```python
from build123d import *

# Parameters (mm, degrees)
RESSALTO_EXTRUS_O1_DEPTH = 15
ESBO_O2_R                = 2.5
CORTE_EXTRUS_O1_DEPTH    = 126.770027202
ESBO_O3_R                = 2.5
CORTE_EXTRUS_O2_DEPTH    = 35.768628391


with BuildPart() as part:
    # Esboço1 → Ressalto-extrusão1 (new body)
    with BuildSketch(Plane.XY):
        with BuildLine():
            Line((98.783276764, -3.569201676), (98.783276764, 17.230798324))
            ThreePointArc((98.783276764, 17.230798324), (99.369063202, 18.645011887), (100.783276764, 19.230798324))
            Line((100.783276764, 19.230798324), (121.583276764, 19.230798324))
            ThreePointArc((121.583276764, 19.230798324), (122.290383546, 19.523691543), (122.583276764, 20.230798324))
            Line((122.583276764, 20.230798324), (122.583276764, 20.430798324))
            Line((122.583276764, 20.430798324), (97.583276764, 20.430798324))
            Line((97.583276764, 20.430798324), (97.583276764, -4.569201676))
            Line((97.583276764, -4.569201676), (97.783276764, -4.569201676))
            ThreePointArc((97.783276764, -4.569201676), (98.490383546, -4.276308457), (98.783276764, -3.569201676))
        make_face()
    extrude(amount=RESSALTO_EXTRUS_O1_DEPTH)

    # Esboço2 → Corte-extrusão1 (cut, through all)
    with BuildSketch(Plane.XZ.offset(-19.230798324)):
        with Locations(Location((111.183276764, 7.5, 0), (0, 0, 270))):
            Circle(ESBO_O2_R)
    extrude(amount=-CORTE_EXTRUS_O1_DEPTH, mode=Mode.SUBTRACT)

    # Esboço3 → Corte-extrusão2 (cut, through all)
    with BuildSketch(Plane(origin=(98.783276764, 0, 0), x_dir=(0, 0, -1), z_dir=(1, 0, 0))):
        with Locations(Location((-7.5, 6.830798324, 0), (0, 0, 90))):
            Circle(ESBO_O3_R)
    extrude(amount=-CORTE_EXTRUS_O2_DEPTH, mode=Mode.SUBTRACT)


solid = part.part
```
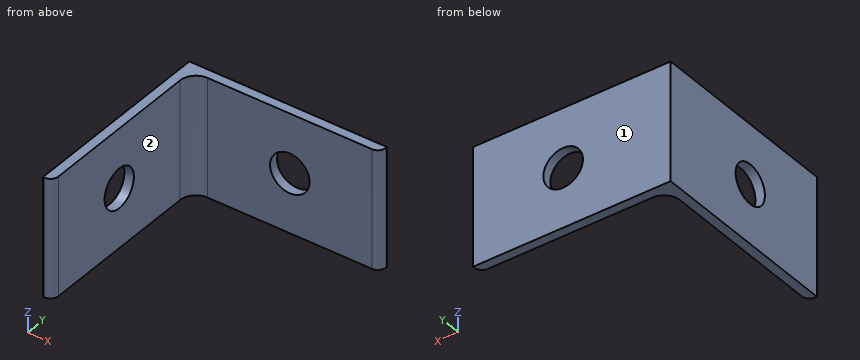
Model file for the job. Use its own axes, mm. Face numbers are marked on the shaded views. A direction names the side the tool comes from. Give positions to 0.01 mm unless a question says otherwise; leave off trailing zeros. Write each loop counter-clockwise with the first axis right and the second up, starting at its lowest first coordinate (ties: lowest second). Pieces come first, ordered by that corner, then holes. Notation, with made-up numbers: M -8,33 L 41,33 A19 ccw 41,52 Z; hole C 48,54.5 d4. An arc over 180 degrees is marked long. Use a Markdown table: item, result.
1) Tool access for the marked faces 1 and 2: list every direction of +Z, -Z, +X, -X, +Y, -Y with a clear straight run to the whole face (end or side of a thin tool).
Responses:
| item | result |
|---|---|
| face 1 | +Z, -Z, +X, -X, +Y |
| face 2 | +Z, -Z, +X, -Y |
2) Drill centre lines: line 1 (Y direction, x = 104.75, z = 8.75); line 2 (X direction, y = 9.75, z = 10.75); line 3 (X direction, y = 19.6, z = 7.5). Where is each one in solid material? Low to high. Write a range as from..to.
Responses:
| item | result |
|---|---|
| line 1 | y = 19.23..20.43 |
| line 2 | x = 97.58..98.78 |
| line 3 | x = 97.58..108.68, 113.68..122.36 |
3) Pin check, flat tips, straight feed: pin 1 (4.5 mm diameter, centred on x = 111.18, z = 7.5, fed in from +Y); pin 2 (6.5 mm diameter, centred on y = 6.83, z = 7.5, fed in from +X). Stop position of each tip, or through.
Responses:
| item | result |
|---|---|
| pin 1 | passes through |
| pin 2 | stops at x = 98.78 |
4) Cut at B-B (z = 1.5). List the corners of the cut face in (x, y).
Responses:
| item | result |
|---|---|
| outline | M 97.58,-4.57 L 97.78,-4.57 A1 ccw 98.78,-3.57 L 98.78,17.23 A2 cw 100.78,19.23 L 121.58,19.23 A1 ccw 122.58,20.23 L 122.58,20.43 L 97.58,20.43 Z |
5) Cut at D-D (y = 14). List the corners of the cut face in (x, z), and give its area (3 significant figures).
Responses:
| item | result |
|---|---|
| outline | M 97.58,0 L 98.78,0 L 98.78,15 L 97.58,15 Z |
| area | 18.0 mm2 |
6) Cut at C-C (z = 5.75). List the corners of the cut face in (x, y).
Responses:
| item | result |
|---|---|
| outline | M 97.58,-4.57 L 97.78,-4.57 A1 ccw 98.78,-3.57 L 98.78,5.05 L 97.58,5.05 Z; M 97.58,8.62 L 98.78,8.62 L 98.78,17.23 A2 cw 100.78,19.23 L 109.4,19.23 L 109.4,20.43 L 97.58,20.43 Z; M 112.97,19.23 L 121.58,19.23 A1 ccw 122.58,20.23 L 122.58,20.43 L 112.97,20.43 Z |
7) Cut at A-A (z = 7.5). List the corners of the cut face in (x, y), and give its area (3 significant figures).
Responses:
| item | result |
|---|---|
| outline | M 97.58,-4.57 L 97.78,-4.57 A1 ccw 98.78,-3.57 L 98.78,4.33 L 97.58,4.33 Z; M 97.58,9.33 L 98.78,9.33 L 98.78,17.23 A2 cw 100.78,19.23 L 108.68,19.23 L 108.68,20.43 L 97.58,20.43 Z; M 113.68,19.23 L 121.58,19.23 A1 ccw 122.58,20.23 L 122.58,20.43 L 113.68,20.43 Z |
| area | 47.0 mm2 |
